from build123d import *

# Parameters (mm, degrees)
SKETCH1_W           = 475
SKETCH1_H           = 250
BOSS_EXTRUDE1_DEPTH = 10
SKETCH2_R           = 2.5
CUT_EXTRUDE1_DEPTH  = 269.572615879
SKETCH3_R           = 2.5
CUT_EXTRUDE2_DEPTH  = 269.572615879
SKETCH4_R           = 5
SKETCH4_W           = 22
SKETCH4_H           = 26
CUT_EXTRUDE3_DEPTH  = 269.572615879


with BuildPart() as part:
    # Sketch1 → Boss-Extrude1 (new body)
    with BuildSketch(Plane.XY):
        Rectangle(SKETCH1_W, SKETCH1_H)
    extrude(amount=BOSS_EXTRUDE1_DEPTH)

    # Sketch2 → Cut-Extrude1 (cut, through all)
    with BuildSketch(Plane.XY.offset(10)):
        with Locations((-207.5, -117.5)):
            Circle(SKETCH2_R)
        with Locations((207.5, -117.5)):
            Circle(SKETCH2_R)
        with Locations((197.5, -117.5)):
            Circle(SKETCH2_R)
        with Locations((-197.5, -117.5)):
            Circle(SKETCH2_R)
    extrude(amount=-CUT_EXTRUDE1_DEPTH, mode=Mode.SUBTRACT)

    # Sketch3 → Cut-Extrude2 (cut, through all)
    with BuildSketch(Plane(origin=(0, 0, 0), x_dir=(-1, 0, 0), z_dir=(0, 0, -1))):
        with Locations((232.5, 95)):
            Circle(SKETCH3_R)
        with Locations((232.5, 85)):
            Circle(SKETCH3_R)
        with Locations((232.5, -85)):
            Circle(SKETCH3_R)
        with Locations((232.5, -95)):
            Circle(SKETCH3_R)
        with Locations((-232.5, 95)):
            Circle(SKETCH3_R)
        with Locations((-232.5, 85)):
            Circle(SKETCH3_R)
        with Locations((-232.5, -85)):
            Circle(SKETCH3_R)
        with Locations((-232.5, -95)):
            Circle(SKETCH3_R)
    extrude(amount=-CUT_EXTRUDE2_DEPTH, mode=Mode.SUBTRACT)

    # Sketch4 → Cut-Extrude3 (cut, through all)
    with BuildSketch(Plane(origin=(0, 0, 0), x_dir=(-1, 0, 0), z_dir=(0, 0, -1))):
        with Locations((156.5, -75)):
            Circle(SKETCH4_R)
        with Locations((126.5, -75)):
            Rectangle(SKETCH4_W, SKETCH4_H)
    extrude(amount=-CUT_EXTRUDE3_DEPTH, mode=Mode.SUBTRACT)


solid = part.part
Part model, mm, in its own coordinate system. A direction names the side the tool comes from. Give positions to 0.01 mm unless a question says otherwise; leave off trailing zeros. Order: outer loops, then holes, each group sorted by start corner. A loop starts at its lowest first (then second) coordinate and runs counter-clockwise, first axis right, second up. Notation, with made-up numbers: (-16.5, 14) - (35.5, 14) arc R18 ccw to (35.5, 47) - close; hole circle Ø8 at (8, 60). An arc over 180 degrees is marked (long way). One line per question, with ' | ' between items.
1. Band-saw the part on B-B on y = -75. List the corners of the cut face in (x, z).
Filled in:
outline: (-237.5, 0) - (-161.5, 0) - (-161.5, 10) - (-237.5, 10) - close; (-151.5, 0) - (-137.5, 0) - (-137.5, 10) - (-151.5, 10) - close; (-115.5, 0) - (237.5, 0) - (237.5, 10) - (-115.5, 10) - close
2. Pull direction Y, two halves, no side cores. Call faces 3 (the face through (-3, -125, 5)), 4 (the face through (237.5, -2, 5)), 5 (the face through (-137.5, -75, 5)): +Y half, -Y half, draft (parallel to the pull), parting line (faces both ways), or undercut.
Filled in:
face 3: -Y half | face 4: draft | face 5: undercut
3. Drill centre lines: probe 1 along Y at (x, z) = (232.5, 5.25); probe 2 along Y at (x, z) = (-156.5, 2.75); probe 3 along Y at (x, z) = (-135, 2). Where is each one in solid material? Low to high.
Filled in:
probe 1: -125 to -97.5, -92.5 to -87.5, -82.5 to 82.5, 87.5 to 92.5, 97.5 to 125 | probe 2: -125 to -80, -70 to 125 | probe 3: -125 to -88, -62 to 125
4. Which spindle directions (+Z, -Z, +X, -X, +Y, -Y) get a long thin tool onto all of the face, cutting with end or side? Do faces 1 (the face through (-3, 2, 0)), 2 (the face through (-126, -88, 5)). Say none if no direction does.
Filled in:
face 1: -Z, +X, -X, +Y, -Y | face 2: +Z, -Z
5. Drop flat-ended pins along their axis: P1, Ø6, axis at x = 232.5, y = 95, coming from the -Z side; P2, Ø4, axis at x = -232.5, y = 95, coming from the -Z side. Give the stop position or say it passes through.
Filled in:
P1: z = 0 | P2: through
6. Band-saw the part on A-A on x = -156.5. List the corners of the cut face in (y, z).
Filled in:
outline: (-125, 0) - (-80, 0) - (-80, 10) - (-125, 10) - close; (-70, 0) - (125, 0) - (125, 10) - (-70, 10) - close
